Here's how the part is built. I have some questions about the finished solid (model axes, mm). Face numbers are marked on the shaded views. A direction names the side the tool comes from. Coordinates: 2 decimals unless noted, no trailing zeros. Order: outer loops, then holes, each group sorted by start corner. A loop starts at its lowest first (then second) coordinate and runs counter-clockwise, first axis right, second up.
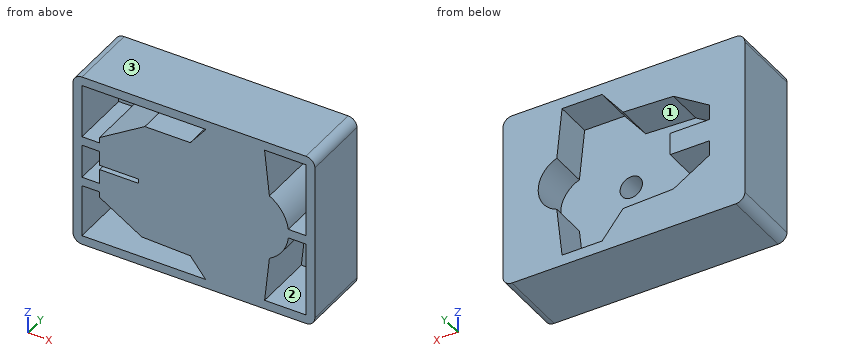
```python
from build123d import *

# Parameters (mm, degrees)
SKETCH1_W              = 54
SKETCH1_H              = 39.25
BOSS_EXTRUDE1_DEPTH    = 15.5
FILLET1_R              = 2
FILLET2_R              = 2
M3_A_START             = -3.329776532
M3_A_BLANK_DEPTH       = 9
M3_A_START_2           = -9.329776532
M3_A_BLANK_2_OUTLINE_R = 2.5
M3_A_BLANK_2_DEPTH     = 6
BODY_MOVE_COPY6_ANGLE  = 90
CUT_EXTRUDE1_DEPTH     = 13.5


with BuildPart() as part:
    # Sketch1 → Boss-Extrude1 (new body)
    with BuildSketch(Plane(origin=(0, 0, 0), x_dir=(1, 0, 0), z_dir=(0, 1, 0))):
        with Locations((27, 19.625)):
            Rectangle(SKETCH1_W, SKETCH1_H)
    extrude(amount=BOSS_EXTRUDE1_DEPTH)

    # Fillet1
    fillet1_edges = [part.edges().sort_by_distance(p)[0] for p in [
        (0, 7.75, 0),
    ]]
    fillet(fillet1_edges, radius=FILLET1_R)

    # Fillet2
    fillet2_edges = [part.edges().sort_by_distance(p)[0] for p in [
        (0, 7.75, -39.25),
        (54, 7.75, -39.25),
        (54, 7.75, 0),
    ]]
    fillet(fillet2_edges, radius=FILLET2_R)


with BuildPart() as body_2:
    # M3-A Blank: read off the stored shape, not the designer's step
    # M3-A Blank outline → M3-A Blank (new body)
    with BuildSketch(Plane(origin=(0, 0, 0), x_dir=(1, 0, 0), z_dir=(0, 1, 0)).offset(M3_A_START)):
        with BuildLine():
            Line((-41.581939277, 43.861919588), (-30.381939277, 42.692718591))
            ThreePointArc((-30.381939277, 42.692718591), (-24.381939277, 38.532817401), (-18.381939277, 42.692718591))
            Line((-18.381939277, 42.692718591), (-7.181939277, 43.861919588))
            Line((-7.181939277, 43.861919588), (-7.181939277, 52.808848959))
            Line((-7.181939277, 52.808848959), (-13.057281533, 57.485652948))
            Line((-13.057281533, 57.485652948), (-13.463960141, 68.720149487))
            Line((-13.463960141, 68.720149487), (-18.39493826, 76.75205199))
            Line((-18.39493826, 76.75205199), (-21.79493826, 76.75205199))
            Line((-21.79493826, 76.75205199), (-21.79493826, 68.00205199))
            Line((-21.79493826, 68.00205199), (-26.79493826, 68.00205199))
            Line((-26.79493826, 68.00205199), (-26.79493826, 76.75205199))
            Line((-26.79493826, 76.75205199), (-30.19493826, 76.75205199))
            Line((-30.19493826, 76.75205199), (-35.227586031, 68.720149487))
            Line((-35.227586031, 68.720149487), (-35.685099465, 57.485652948))
            Line((-35.685099465, 57.485652948), (-41.581939277, 52.808848959))
            Line((-41.581939277, 52.808848959), (-41.581939277, 43.861919588))
        make_face()
    extrude(amount=M3_A_BLANK_DEPTH)

    # M3-A Blank 2 outline → M3-A Blank 2 (add)
    with BuildSketch(Plane(origin=(0, 0, 0), x_dir=(1, 0, 0), z_dir=(0, 1, 0)).offset(M3_A_START_2)):
        with Locations((-24.335480832, 54.269355582)):
            Circle(M3_A_BLANK_2_OUTLINE_R)
    extrude(amount=M3_A_BLANK_2_DEPTH)


with BuildPart() as body_2_1:
    # Body-Move/Copy4: moved
    add(body_2.part.moved(Location((42.5, 8.919688157, 37.96700657))))


with BuildPart() as body_2_2:
    # Body-Move/Copy5: moved
    add(body_2_1.part.moved(Location((8.915108254, 0, 0))))


with BuildPart() as body_2_3:
    # Body-Move/Copy6: moved
    add(body_2_2.part.rotate(Axis((27.033168977, 0, -19.675428126), (0, 1, 0)), BODY_MOVE_COPY6_ANGLE))


with BuildPart() as body_2_4:
    # Body-Move/Copy7: moved
    add(body_2_3.part.moved(Location((0, 1.103676274, 0))))


with BuildPart() as body_2_5:
    # Body-Move/Copy8: moved
    add(body_2_4.part.moved(Location((0, 0.5, 0))))


with BuildPart() as part_1:
    add(part.part)

    # Intersect1: read off the stored shape, not the designer's step
    # Intersect1: cut body 2
    add(body_2_5.part, mode=Mode.SUBTRACT)

    # Sketch3 → Cut-Extrude1 (cut)
    with BuildSketch(Plane(origin=(0, 0, 0), x_dir=(-1, 0, 0), z_dir=(0, -1, 0))):
        Polygon((-5.923551682, 12.755419679), (-16.048628272, 6.41122612), (-26.192603819, 6.41122612), (-29.691162465, 2), (-2, 2), (-2, 14.017695962), (-5.923551682, 14.017695962), align=None)
        Polygon((-2, 37.25), (-29.60864948, 37.25), (-26.198159594, 32.965493874), (-15.357384062, 32.57306761), (-5.923551682, 26.781411023), (-5.923551682, 25.507817982), (-2, 25.507817982), align=None)
        Polygon((-5.923551682, 20.262429143), (-14.673551682, 20.262429143), (-14.673551682, 19.262429143), (-5.923551682, 19.262429143), (-5.923551682, 16.008924411), (-2, 16.008924411), (-2, 23.521920083), (-5.923551682, 23.521920083), align=None)
        with BuildLine():
            Line((-42.774921098, 2), (-52, 2))
            Line((-52, 2), (-52, 18.627764364))
            Line((-52, 18.627764364), (-48.077251764, 18.627764364))
            ThreePointArc((-48.077251764, 18.627764364), (-46.712904885, 14.985289801), (-43.85505184, 12.346778986))
            Line((-43.85505184, 12.346778986), (-42.774921098, 2))
        make_face()
        with BuildLine():
            Line((-52, 37.25), (-42.78544978, 37.25))
            Line((-42.78544978, 37.25), (-43.85505184, 27.004077266))
            ThreePointArc((-43.85505184, 27.004077266), (-46.741831066, 24.322246322), (-48.089593706, 20.619646239))
            Line((-48.089593706, 20.619646239), (-52, 20.619646239))
            Line((-52, 20.619646239), (-52, 37.25))
        make_face()
    extrude(amount=-CUT_EXTRUDE1_DEPTH, mode=Mode.SUBTRACT)


solid = part_1.part
```
Q1. If we section it at D-D on x = 37: Write out the boundary of the cut face in (y, z).
Q2. If we section it at C-C on z = -9.5: Write out the boundary of the cut face in (x, y).
Q3. If we section it at A-A on x = 4.5: Write out the boundary of the cut face in (y, z).
Q4. I need wall thicknesses on L1, parallel to Z at x = 50, y = 7; L2, parallel to Z at x = 33, y = 7.25; L3, parallel to X at y = 8.25, z = -36. Which ranges of each line are inside material? Lowest first, please.
Q5. For the marked faces 1, 2 and 3, which set-ups out of +Z, -Z, +X, -X, +Y, -Y let a thin tool reach every point of the face, with its end or its side?
Q6. Will this pin go through, and if not, where does the flat tip stop? pin 1 (2.5 mm diameter, centred on x = 31, z = -19.5, fed in from +Y).
Q7. If we section it at B-B on y = 9.5: Give the number of separate pieces and of enclosed holes in the cut face, then the cut area to 3 significant figures.
Reply:
1. outline: (0, -39.25) - (15.5, -39.25) - (15.5, -36.88) - (7.19, -36.88) - (7.19, -2.48) - (15.5, -2.48) - (15.5, 0) - (0, 0) - close
2. outline: (0, 0) - (2, 0) - (2, 13.5) - (11.12, 13.5) - (11.12, 0) - (43.56, 0) - (43.56, 13.5) - (52, 13.5) - (52, 0) - (54, 0) - (54, 15.5) - (41.55, 15.5) - (41.55, 7.19) - (14.89, 7.19) - (14.89, 15.5) - (0, 15.5) - close
3. outline: (0, -39.25) - (15.5, -39.25) - (15.5, 0) - (0, 0) - (0, -2) - (13.5, -2) - (13.5, -14.02) - (0, -14.02) - (0, -16.01) - (13.5, -16.01) - (13.5, -23.52) - (0, -23.52) - (0, -25.51) - (13.5, -25.51) - (13.5, -37.25) - (0, -37.25) - close
4. L1: z = -39.25 to -37.25, -20.62 to -18.63, -2 to 0
4. L2: z = -39.25 to -36.88, -2.48 to 0
4. L3: x = 0 to 2, 28.61 to 31.17, 40.91 to 42.92, 52 to 54
5. face 1: +Y
5. face 2: -Y
5. face 3: +Z, +X, -X, +Y, -Y
6. pin 1: stops at y = 1.19
7. separate pieces: 1
7. enclosed holes: 6
7. area: 637 mm2
